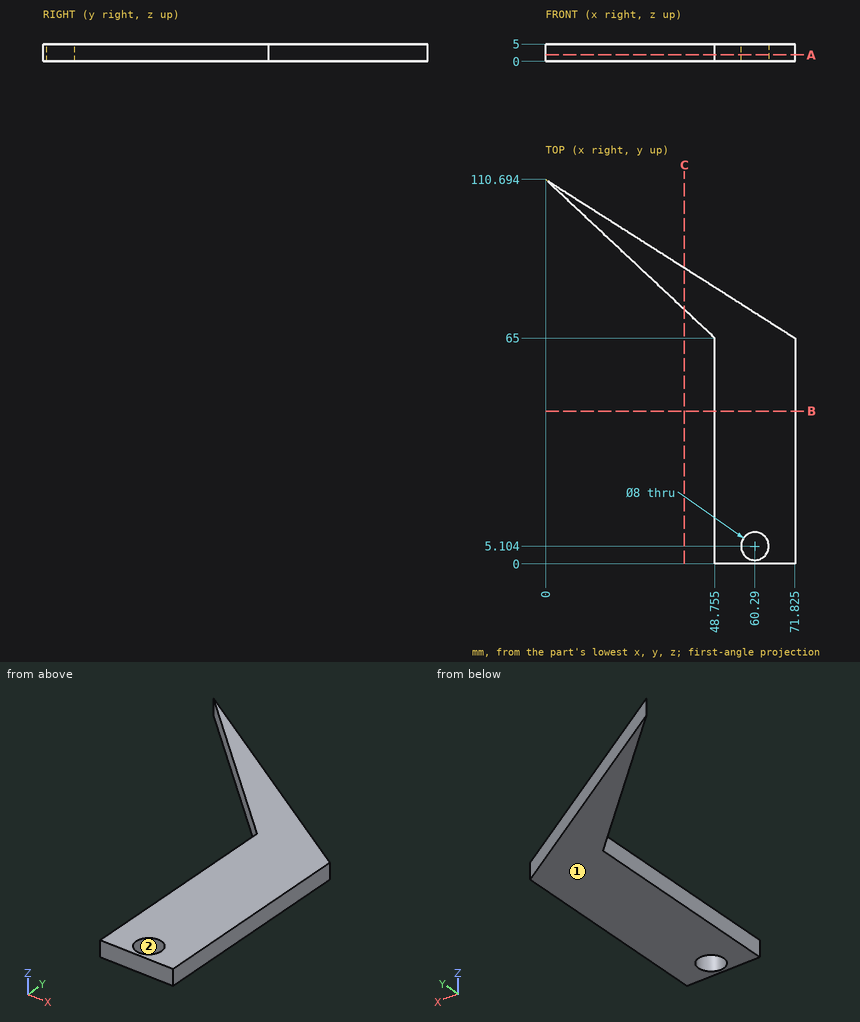
The drawing under review shows one solid part. Ordinate dimensions are in mm from its lowest x, y, z. Round coordinates to 2 decimals unless told otherwise and drop trailing zeros. Order: outer loops, then holes, each group sorted by start corner. A loop starts at its lowest first (then second) coordinate and runs counter-clockwise, first axis right, second up. Notation, with made-up numbers: (-24, -7.5) -> (-12, -7.5) arc R28 ccw to (-12, 28.5) -> close; hole circle Ø7 at (84.5, 69). An arc over 180 degrees is marked (long way). Return JSON: item names as keys, results as strings.
1. The part is to be moulded in two halves that separate along X. For the marked faces 1 and 2, say which applies: +X half, -X half, draft (parallel to the pull), parting line (faces both ways), or undercut.
Answer block:
{"face 1": "draft", "face 2": "undercut"}
2. For L1, parallel to X at y = 40.5, z = 1.6 (1 decimal); L2, parallel to X at y = 7.5, z = 3 (1 decimal); L3, parallel to X at y = 6, z = 2.6 (1 decimal), list the stretches that pass through material, from the lowest coordinate up. Write a range as [from, to].
Answer block:
{"L1": "x = [48.8, 71.8]", "L2": "x = [48.8, 57.1], [63.5, 71.8]", "L3": "x = [48.8, 56.4], [64.2, 71.8]"}
3. Insertion check: P1, Ø10, axis at x = 41, y = 62.5, coming from the +Z side. The pin has a flat end and moves straight along its axis. Give the tip position at first contact, or say it passes through.
Answer block:
{"P1": "passes through"}
4. Take a section at C-C (x = 40). Write out the cut boundary in (y, z) (1 decimal), then the cut area to 3 significant figures.
Answer block:
{"outline": "(73.2, 0) -> (85.2, 0) -> (85.2, 5) -> (73.2, 5) -> close", "area": "60.2 mm²"}
5. Take a section at B-B (y = 44). Write out the cut boundary in (x, z) (1 decimal).
Answer block:
{"outline": "(48.8, 0) -> (71.8, 0) -> (71.8, 5) -> (48.8, 5) -> close"}
6. Take a section at A-A (z = 1.9). Write out the cut boundary in (x, y) (1 decimal).
Answer block:
{"outline": "(0, 110.7) -> (48.8, 65) -> (48.8, 0) -> (71.8, 0) -> (71.8, 65) -> close; hole circle Ø8 at (60.3, 5.1)"}
